Design review of the part shown in the three views and the two pictorial views. Dimensions are in mm from the part's minimum x, y and z. Round coordinates to 2 decimals unless told otherwise and drop trailing zeros. Loops run counter-clockwise (first coordinate to the right, second up) from the corner with the lowest first, then second, coordinate; pieces in that order, holes last. Notation, with made-up numbers: M 10.5,34.5 L 40.5,34.5 A22 ccw 40.5,63.5 Z; hole C -26,46.25 d2. An arc over 180 degrees is marked long. One line per question, with ' | ' between items.
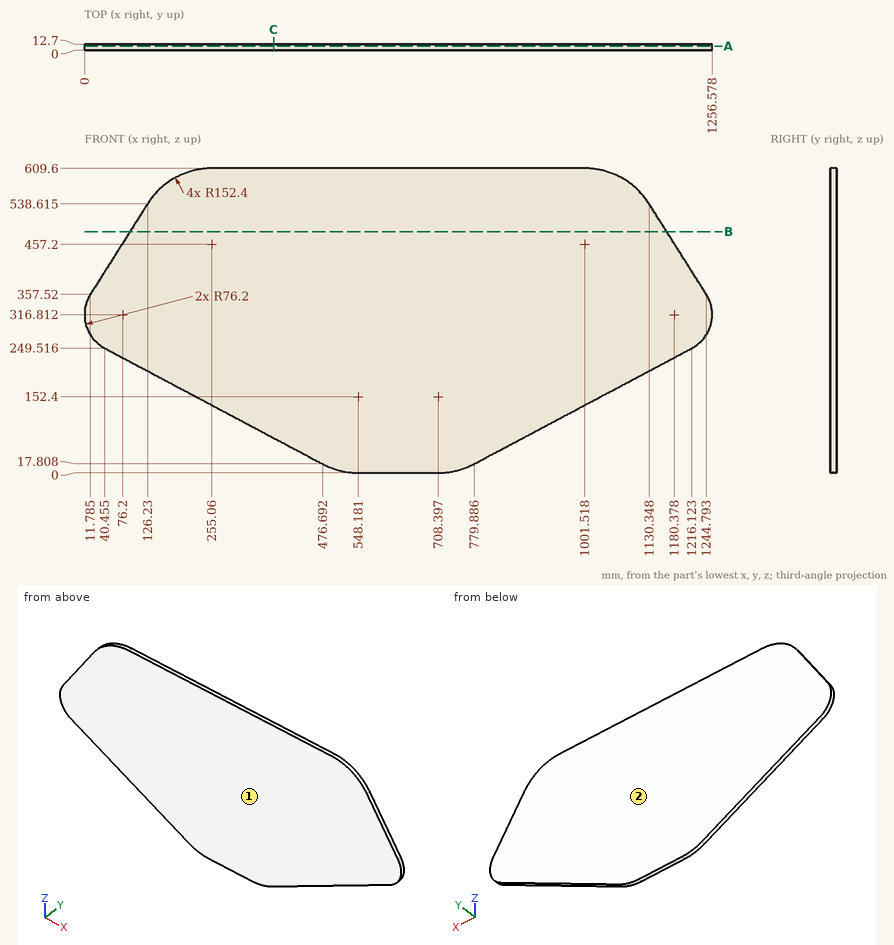
1) For line 1 (X direction, y = 4.75, z = 74.5) (1 decimal); line 2 (Z direction, x = 367, y = 11.25); line 3 (X direction, y = 5.5, z = 565) (1 decimal), list the stretches that pass through material, from the lowest coordinate up.
Output values:
line 1: x = 370 to 886.6 | line 2: z = 76.07 to 609.6 | line 3: x = 147.3 to 1109.2
2) Add section B-B on z = 483. State the section outline as (x, y) points (1 decimal).
Output values:
outline: M 91.1,0 L 1165.5,0 L 1165.5,12.7 L 91.1,12.7 Z
3) Add section C-C on x = 378.5. State the section outline as (y, z) points, then the cut area to 3 significant figures.
Output values:
outline: M 0,69.96 L 12.7,69.96 L 12.7,609.6 L 0,609.6 Z | area: 6,850 mm²
4) Mouldability with a two-part tool opening along Y and no side actions: class the marked faces 1 and 2 as +Y half, -Y half, draft (parallel to the pull), parting line (faces both ways), or undercut.
Output values:
face 1: -Y half | face 2: +Y half
5) Insertion check: P1, Ø1.5, axis at x = 152.5, y = 8.5, coming from the -Z side (1 decimal); P2, Ø2, axis at y = 11.5, z = 506.5, coming from the -X side; P3, Ø4, axis at y = 10.5, z = 312.5, coming from the +X side. Each pin has a flat end and moves straight along its axis. Give the tip position at first contact, or say it passes through.
Output values:
P1: stops at z = 189.6 | P2: stops at x = 105.3 | P3: stops at x = 1256.54
6) Add section A-A on y = 8.5. State the section outline as (x, z) points (1 decimal).
Output values:
outline: M 11.8,357.5 A76.2 ccw 40.5,249.5 L 476.7,17.8 A152.4 ccw 548.2,0 L 708.4,0 A152.4 ccw 779.9,17.8 L 1216.1,249.5 A76.2 ccw 1244.8,357.5 L 1130.3,538.6 A152.4 ccw 1001.5,609.6 L 255.1,609.6 A152.4 ccw 126.2,538.6 Z
